Design review of the part built by this model. Coordinates are the model's own, in mm. A direction names the side the tool comes from. Give positions to 0.01 mm unless a question says otherwise; leave off trailing zeros. Order: outer loops, then holes, each group sorted by start corner. A loop starts at its lowest first (then second) coordinate and runs counter-clockwise, first axis right, second up. Notation, with made-up numbers: M 39.25,-2.75 L 82.25,-2.75 A29 ccw 82.25,17.25 Z; hole C 24,8.5 d10. An arc over 180 degrees is marked long. Answer as a JSON object with one key per item and string values.
from build123d import *

# Parameters (mm, degrees)
SKETCH1_R           = 14.5
BOSS_EXTRUDE1_DEPTH = 4
SKETCH2_W           = 2
SKETCH2_H           = 3
BOSS_EXTRUDE2_DEPTH = 33.973847717
SKETCH3_W           = 3
SKETCH3_H           = 6
BOSS_EXTRUDE3_DEPTH = 2
CUT_EXTRUDE1_REACH  = 45.684
SKETCH5_W           = 3
SKETCH5_H           = 6
BOSS_EXTRUDE4_DEPTH = 2
CUT_EXTRUDE2_REACH  = 45.684
FILLET1_R           = 1
FILLET2_R           = 0.5


with BuildPart() as part:
    # Sketch1 → Boss-Extrude1 (new body)
    with BuildSketch(Plane(origin=(0, 0, 0), x_dir=(0, 1, 0), z_dir=(0, 0, 1))):
        with Locations(Location((0, 0, 0), (0, 0, 270))):
            Circle(SKETCH1_R)
    extrude(amount=BOSS_EXTRUDE1_DEPTH)

    # Sketch2 → Boss-Extrude2 (add)
    with BuildSketch(Plane.XY.offset(4)):
        with Locations((-11.353510083, 0)):
            Rectangle(SKETCH2_W, SKETCH2_H)
        with Locations((11.353510083, 0)):
            Rectangle(SKETCH2_W, SKETCH2_H)
    extrude(amount=BOSS_EXTRUDE2_DEPTH)

    # Sketch3 → Boss-Extrude3 (add)
    with BuildSketch(Plane(origin=(-12.353510083, 0, 0), x_dir=(0, -1, 0), z_dir=(-1, 0, 0))):
        with Locations((0, 34.973847717)):
            Rectangle(SKETCH3_W, SKETCH3_H)
    extrude(amount=BOSS_EXTRUDE3_DEPTH)

    # Sketch4 → Cut-Extrude1 (cut, up to next)
    with BuildSketch(Plane.XZ.offset(1.5), mode=Mode.PRIVATE) as cut_extrude1_sk1:
        Polygon((-12.353510083, 31.973847717), (-14.353510083, 33.973847717), (-14.353510083, 31.973847717), align=None)
    cut_extrude1_tool1 = extrude(cut_extrude1_sk1.sketch, amount=-CUT_EXTRUDE1_REACH, mode=Mode.PRIVATE) & part.part
    # Sketch4 → Cut-Extrude1 (cut, up to next)
    with BuildSketch(Plane.XZ.offset(1.5), mode=Mode.PRIVATE) as cut_extrude1_sk2:
        Polygon((-12.353510083, 37.973847717), (-14.353510083, 35.973847717), (-14.353510083, 37.973847717), align=None)
    cut_extrude1_tool2 = extrude(cut_extrude1_sk2.sketch, amount=-CUT_EXTRUDE1_REACH, mode=Mode.PRIVATE) & part.part
    add(cut_extrude1_tool1.solids().sort_by_distance((-13.686843, -1.5, 32.640514))[0], mode=Mode.SUBTRACT)
    add(cut_extrude1_tool2.solids().sort_by_distance((-13.686843, -1.5, 37.307181))[0], mode=Mode.SUBTRACT)

    # Sketch5 → Boss-Extrude4 (add)
    with BuildSketch(Plane.YZ.offset(12.353510083)):
        with Locations((0, 34.973847717)):
            Rectangle(SKETCH5_W, SKETCH5_H)
    extrude(amount=BOSS_EXTRUDE4_DEPTH)

    # Sketch6 → Cut-Extrude2 (cut, up to next)
    with BuildSketch(Plane.XZ.offset(1.5), mode=Mode.PRIVATE) as cut_extrude2_sk1:
        Polygon((12.353510083, 31.973847717), (14.353510083, 33.973847717), (14.353510083, 31.973847717), align=None)
    cut_extrude2_tool1 = extrude(cut_extrude2_sk1.sketch, amount=-CUT_EXTRUDE2_REACH, mode=Mode.PRIVATE) & part.part
    # Sketch6 → Cut-Extrude2 (cut, up to next)
    with BuildSketch(Plane.XZ.offset(1.5), mode=Mode.PRIVATE) as cut_extrude2_sk2:
        Polygon((12.353510083, 37.973847717), (14.353510083, 35.973847717), (14.353510083, 37.973847717), align=None)
    cut_extrude2_tool2 = extrude(cut_extrude2_sk2.sketch, amount=-CUT_EXTRUDE2_REACH, mode=Mode.PRIVATE) & part.part
    add(cut_extrude2_tool1.solids().sort_by_distance((13.686843, -1.5, 32.640514))[0], mode=Mode.SUBTRACT)
    add(cut_extrude2_tool2.solids().sort_by_distance((13.686843, -1.5, 37.307181))[0], mode=Mode.SUBTRACT)

    # Fillet1
    fillet1_edges = [part.edges().sort_by_distance(p)[0] for p in [
        (-12.353510083, 0, 4),
        (-11.353510083, -1.5, 4),
        (12.353510083, 0, 4),
        (11.353510083, 1.5, 4),
        (10.353510083, 0, 4),
        (11.353510083, -1.5, 4),
        (-10.353510083, 0, 4),
        (-11.353510083, 1.5, 4),
    ]]
    fillet(fillet1_edges, radius=FILLET1_R)

    # Fillet2
    fillet2_edges = [part.edges().sort_by_distance(p)[0] for p in [
        (-10.353510083, 0, 37.973847717),
        (10.353510083, 0, 37.973847717),
        (-12.353510083, 0, 31.973847717),
        (-14.353510083, 0, 33.973847717),
        (-12.353510083, 0, 37.973847717),
        (-14.353510083, 0, 35.973847717),
        (12.353510083, 0, 31.973847717),
        (14.353510083, 0, 33.973847717),
        (12.353510083, 0, 37.973847717),
        (14.353510083, 0, 35.973847717),
    ]]
    fillet(fillet2_edges, radius=FILLET2_R)


solid = part.part
(1) We need section C-C (x = 0). Write out the cut boundary in (y, z), plus the area to 3 significant figures.
Checked values:
{"outline": "M -14.5,0 L 14.5,0 L 14.5,4 L -14.5,4 Z", "area": "116 mm^2"}
(2) We need section D-D (x = -11.5). Write out the cut boundary in (y, z), plus the area to 3 significant figures.
Checked values:
{"outline": "M -8.83,0 L 8.83,0 L 8.83,4 L 2.5,4 A1 cw 1.5,5 L 1.5,37.97 L -1.5,37.97 L -1.5,5 A1 cw -2.5,4 L -8.83,4 Z", "area": "173 mm^2"}
(3) To check wall thickness, follow L1, parallel to Z at x = 4.5, y = -9.75; L2, parallel to Y at x = 10.75, z = 36.5; L3, parallel to Z at x = 12, y = -2. State the ranges of each line that lie inside material, in increasing order. Write a range as from..to.
Checked values:
{"L1": "z = 0..4", "L2": "y = -1.5..1.5", "L3": "z = 0..4.13"}
(4) Draft analysis for pull direction X (two halves, no side actions). For faces 1 (the flat face through (14.354, 0, 35)), 2 (the cylindrical face through (-9.918, 0.035, 4.175)), 3 (the flat face through (-13.34, -0.02, 32.96)), state which applies: +X half, -X half, draft (parallel to the pull), parting line (faces both ways), or undercut.
Checked values:
{"face 1": "+X half", "face 2": "undercut", "face 3": "-X half"}
(5) Insertion check: pin 1 (1.2 mm diameter, centred on x = -12.5, z = 26.5, fed in from -Y); pin 2 (3.5 mm diameter, centred on y = -0.5, z = 16.5, fed in from -X); pin 3 (1.5 mm diameter, centred on y = 0, z = 21, fed in from +X). Each pin has a flat end and moves straight along its axis. Give the tip position at first contact, or say it passes through.
Checked values:
{"pin 1": "stops at y = -1.5", "pin 2": "stops at x = -12.35", "pin 3": "stops at x = 12.35"}
(6) We need section A-A (z = 24). Write out the cut boundary in (x, y), plus the area to 3 significant figures.
Checked values:
{"outline": "M -12.35,-1.5 L -10.35,-1.5 L -10.35,1.5 L -12.35,1.5 Z; M 10.35,-1.5 L 12.35,-1.5 L 12.35,1.5 L 10.35,1.5 Z", "area": "12.0 mm^2"}
(7) Tool access review of faces 4 (the cylindrical face through (9.918, 0.035, 4.175)), 5 (the flat face through (11, 1.5, 21)), 6 (the flat face through (-12.354, 0, 18)), 7 (the cylindrical face through (12.789, 0.035, 4.175)), 8 (the flat face through (-14.354, 0, 35)): name each direction out of +Z, -Z, +X, -X, +Y, -Y from which nothing blocks a thin tool from reaching the whole face with its end or side.
Checked values:
{"face 4": "+Z, +Y, -Y", "face 5": "+Z, +X, -X, +Y", "face 6": "-X, +Y, -Y", "face 7": "+X, +Y, -Y", "face 8": "+Z, -X, +Y, -Y"}
